from build123d import *
from build123d.topology import SkipClean

# Parameters (mm, degrees)
SKETCH1_R                = 97
SKETCH1_R_2              = 23.5
BOSS_EXTRUDE1_DEPTH      = 112.5
SKETCH2_R                = 250
SKETCH2_R_2              = 140
CUT_EXTRUDE8_DEPTH       = 80.5
BOSS_EXTRUDE2_START      = -160
SKETCH4_R                = 100
BOSS_EXTRUDE2_DEPTH      = 62.02041
SKETCH5_R                = 10.15
CUT_EXTRUDE9_DEPTH       = 15
SKETCH6_R                = 50
CUT_EXTRUDE10_DEPTH      = 25
BOSS_EXTRUDE3_REACH      = 775.894
BOSS_EXTRUDE3_END_RADIUS = 140
BOSS_EXTRUDE3_START      = -325
SKETCH7_R                = 37.5
SKETCH8_R                = 28.1
CUT_EXTRUDE11_DEPTH      = 310


with BuildPart() as part:
    # Sketch1 → Boss-Extrude1 (new, symmetric)
    with BuildSketch(Plane(origin=(0, 0, 0), x_dir=(1, 0, 0), z_dir=(0, 1, 0))):
        with BuildLine():
            Line((130.766968306, 50), (175, 50))
            ThreePointArc((175, 50), (225, 0), (175, -50))
            Line((175, -50), (130.766968306, -50))
            ThreePointArc((130.766968306, -50), (70, -121.24355653), (-22.082213964, -138.247516529))
            Line((-22.082213964, -138.247516529), (-44.198729811, -176.554445662))
            ThreePointArc((-44.198729811, -176.554445662), (-112.5, -194.855715851), (-130.801270189, -126.554445662))
            Line((-130.801270189, -126.554445662), (-108.684754342, -88.247516529))
            ThreePointArc((-108.684754342, -88.247516529), (-140, 0), (-108.684754342, 88.247516529))
            Line((-108.684754342, 88.247516529), (-130.801270189, 126.554445662))
            ThreePointArc((-130.801270189, 126.554445662), (-112.5, 194.855715851), (-44.198729811, 176.554445662))
            Line((-44.198729811, 176.554445662), (-22.082213964, 138.247516529))
            ThreePointArc((-22.082213964, 138.247516529), (70, 121.24355653), (130.766968306, 50))
        make_face()
        with Locations(Location((0, 0, 0), (0, 0, 270))):
            Circle(SKETCH1_R, mode=Mode.SUBTRACT)
        with Locations(Location((175, 0, 0), (0, 0, 270))):
            Circle(SKETCH1_R_2, mode=Mode.SUBTRACT)
        with Locations(Location((-87.5, -151.554445662, 0), (0, 0, 270))):
            Circle(SKETCH1_R_2, mode=Mode.SUBTRACT)
        with Locations(Location((-87.5, 151.554445662, 0), (0, 0, 270))):
            Circle(SKETCH1_R_2, mode=Mode.SUBTRACT)
    extrude(amount=BOSS_EXTRUDE1_DEPTH, both=True)

    # Sketch2 → Cut-Extrude8 (cut, symmetric)
    with SkipClean():  # the faces are left unmerged after this step: merging them gives an invalid solid
        with BuildSketch(Plane(origin=(0, 0, 0), x_dir=(1, 0, 0), z_dir=(0, 1, 0))):
            Circle(SKETCH2_R)
            with Locations(Location((0, 0, 0), (0, 0, 99.075167572))):
                Circle(SKETCH2_R_2, mode=Mode.SUBTRACT)
        extrude(amount=CUT_EXTRUDE8_DEPTH, both=True, mode=Mode.SUBTRACT)

    # Sketch4 → Boss-Extrude2 (add)
    with SkipClean():  # the faces are left unmerged after this step: merging them gives an invalid solid
        with BuildSketch(Plane(origin=(0, 0, 0), x_dir=(0, 0, -1), z_dir=(1, 0, 0)).offset(BOSS_EXTRUDE2_START)):
            with Locations(Location((0, 0, 0), (0, 0, 180))):
                Circle(SKETCH4_R)
        extrude(amount=BOSS_EXTRUDE2_DEPTH)

    # Sketch5 → Cut-Extrude9 (cut)
    with SkipClean():  # the faces are left unmerged after this step: merging them gives an invalid solid
        with BuildSketch(Plane.ZY.offset(160)):
            with Locations((0, 75)):
                Circle(SKETCH5_R)
            with Locations((64.951905284, -37.5)):
                Circle(SKETCH5_R)
            with Locations((-64.951905284, -37.5)):
                Circle(SKETCH5_R)
        extrude(amount=-CUT_EXTRUDE9_DEPTH, mode=Mode.SUBTRACT)

    # Sketch6 → Cut-Extrude10 (cut)
    with SkipClean():  # the faces are left unmerged after this step: merging them gives an invalid solid
        with BuildSketch(Plane.ZY.offset(160)):
            Circle(SKETCH6_R)
        extrude(amount=-CUT_EXTRUDE10_DEPTH, mode=Mode.SUBTRACT)

    # Boss-Extrude3: up to this cylinder (the profile starts outside it)
    with SkipClean():  # the faces are left unmerged after this step: merging them gives an invalid solid
        boss_extrude3_end = Plane(origin=(0, 0, 0), z_dir=(0, -1, 0)) * Cylinder(BOSS_EXTRUDE3_END_RADIUS, 1832.788, mode=Mode.PRIVATE)
        # Sketch7 → Boss-Extrude3 (add, up to the surface)
        with BuildSketch(Plane.ZY.offset(160).offset(BOSS_EXTRUDE3_START), mode=Mode.PRIVATE) as boss_extrude3_sk1:
            with Locations(Location((0, 0, 0), (0, 0, 180))):
                Circle(SKETCH7_R)
        boss_extrude3_tool1 = extrude(boss_extrude3_sk1.sketch, amount=BOSS_EXTRUDE3_REACH, mode=Mode.PRIVATE) - boss_extrude3_end
        add(boss_extrude3_tool1.solids().sort_by_distance((165, 0, 0))[0])

    # Sketch8 → Cut-Extrude11 (cut)
    with SkipClean():  # the faces are left unmerged after this step: merging them gives an invalid solid
        with BuildSketch(Plane.ZY.offset(160)):
            Circle(SKETCH8_R)
        extrude(amount=-CUT_EXTRUDE11_DEPTH, mode=Mode.SUBTRACT)


solid = part.part
Input: part model. Units: mm. Frame: model coordinates. A direction names the side the tool comes from. Round coordinates to 2 decimals unless told otherwise and drop trailing zeros. Order: outer loops, then holes, each group sorted by start corner. A loop starts at its lowest first (then second) coordinate and runs counter-clockwise, first axis right, second up.
1. Cut plane D-D, the plane z = 0. State how many separate pieces and enclosed holes the cut face has, then the cut area to 3 significant figures.
The answers:
separate pieces: 5
enclosed holes: 0
area: 19,700 mm2
2. Pin query (flat end, axial travel): P1, Ø1.5, axis at y = -64.5, z = -78.5, coming from the -X side; P2, Ø10, axis at y = -40, z = -64, coming from the -X side; P3, Ø9.5, axis at x = 159.5, y = 102, coming from the -Z side. Return the tip coordinate at first contact, or that it passes through.
The answers:
P1: stops at x = -116.43
P2: stops at x = -145
P3: stops at z = -50
3. Material intervals for line 1 (X direction, y = -104.5, z = 0); line 2 (Z direction, x = -87.5, y = -102); line 3 (X direction, y = 60, z = 0), sorted ascending.
The answers:
line 1: x = -140 to -97, 97 to 151.5, 198.5 to 225
line 2: z = -201.55 to -175.05, -128.05 to -41.87, 41.87 to 128.05, 175.05 to 201.55
line 3: x = -160 to -97, 97 to 140
4. Set-up query: faces 4 (the face through (150, 0, 0)), 5 (the face through (153, 97, 50)), 6 (the face through (165, -1, 1)), 7 (the face through (-119.9, 96.72, 107.67)). Return all of +Z, -Z, +X, -X, +Y, -Y with unobstructed straight access to the full face (end or side cutting, diameter ignored); none if empty.
The answers:
face 4: -X
face 5: +Z, +X, +Y, -Y
face 6: +Z, -Z, +X
face 7: -X, +Y
5. Cut plane B-B, the plane z = 81. Output: boundary loops of the cut face in (x, y).
The answers:
outline: (-160, -58.64) - (-114.19, -58.64) - (-114.19, -112.5) - (-53.37, -112.5) - (-53.37, 112.5) - (-114.19, 112.5) - (-114.19, 58.64) - (-160, 58.64) - close; (53.37, -112.5) - (114.19, -112.5) - (114.19, 112.5) - (53.37, 112.5) - close
6. Cut plane A-A, the plane x = 0. Output: boundary loops of the cut face in (y, z), then the cut area to 4 significant figures.
The answers:
outline: (-112.5, -140) - (112.5, -140) - (112.5, -97) - (-112.5, -97) - close; (-112.5, 97) - (112.5, 97) - (112.5, 140) - (-112.5, 140) - close
area: 19,350 mm2
7. Mould query, pull axis Z, two halves, no side actions, for faces 1 (the face through (224.988, -96.276, -1.099)), 2 (the face through (-145, -37, -65)), 3 (the face through (-32.986, 96.724, 157.133)). Classes: released by +Z, released by -Z, zero draft, split by the parting line, or undercut.
The answers:
face 1: split by the parting line
face 2: undercut
face 3: released by +Z
